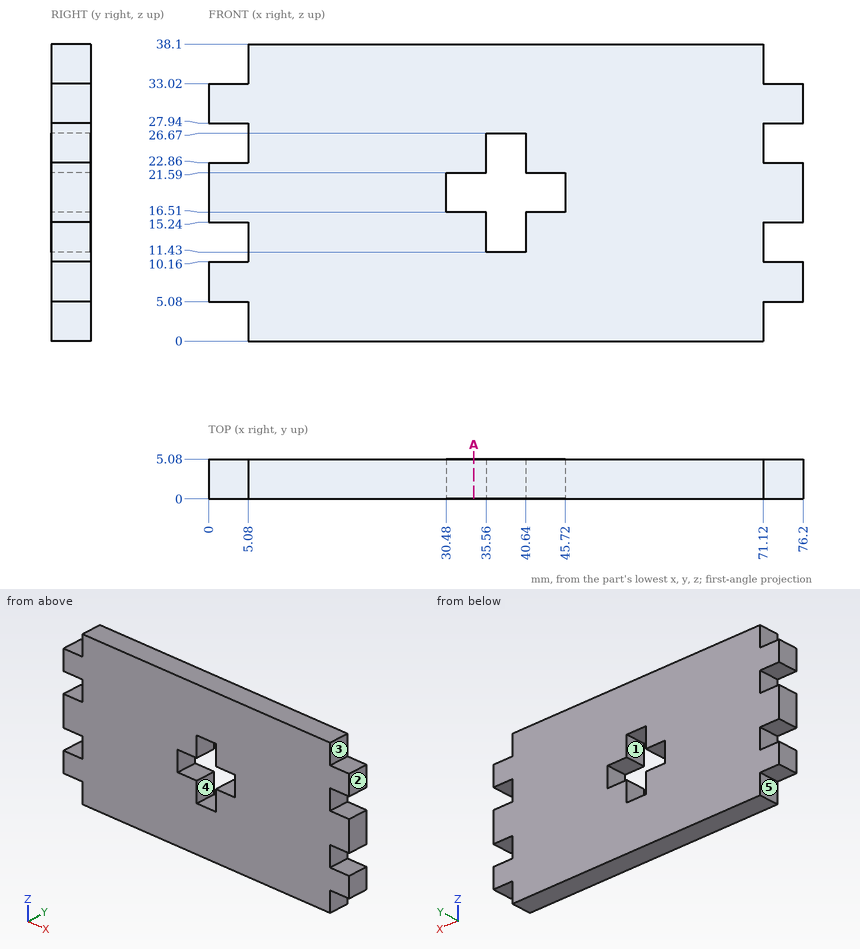
Drawing for the job (mm, zero at the part's lowest x, y, z). A direction names the side the tool comes from. Round coordinates to 2 decimals unless told otherwise and drop trailing zeros. Order: outer loops, then holes, each group sorted by start corner. A loop starts at its lowest first (then second) coordinate and runs counter-clockwise, first axis right, second up. Notation, with made-up numbers: (-18.75, -18.75) -> (-4.75, -18.75) arc R13 ccw to (-4.75, 4.25) -> close; hole circle Ø9 at (29.25, 66). An arc over 180 degrees is marked (long way). Write item = value, one per line. Start each with the question number.
(1) Cut at A-A, the plane x = 34. List the corners of the cut face in (y, z), then the cut area to 3 significant figures.
(2) Pin check, flat tips, straight feed: P1, Ø1.5, axis at y = 3, z = 3.5, coming from the -X side; P2, Ø1.5, axis at y = 1.5, z = 11.5, coming from the +X side; P3, Ø2.5, axis at x = 74, y = 2.5, coming from the -Z side. Stop position of each tip, or through.
(3) Probe line 1 (Z direction, x = 4, y = 3.95); line 2 (X direction, y = 3.5, z = 26); line 3 (X direction, y = 0.4, z = 16). List the from-to ranges inside material, lowest first. Write a range as [from, to].
(4) Pull direction Z, two halves, no side cores. Call the marked faces 4 and 5: released by +Z, released by -Z, zero draft, split by the parting line, or undercut.
(5) Which spindle directions (+Z, -Z, +X, -X, +Y, -Y) get a long thin tool onto all of the face, cutting with end or side? Do the marked faces 1, 2 and 3. Say none if no direction does.
Model answer:
q1.outline = (0, 0) -> (5.08, 0) -> (5.08, 16.51) -> (0, 16.51) -> close; (0, 21.59) -> (5.08, 21.59) -> (5.08, 38.1) -> (0, 38.1) -> close
q1.area = 168 mm2
q2.P1 = 5.08
q2.P2 = 71.12
q2.P3 = 5.08
q3.line_1 = [5.08, 10.16], [15.24, 22.86], [27.94, 33.02]
q3.line_2 = [5.08, 35.56], [40.64, 71.12]
q3.line_3 = [0, 35.56], [40.64, 76.2]
q4.face_4 = undercut
q4.face_5 = zero draft
q5.face_1 = +Y, -Y
q5.face_2 = +Z, -Z, +X, +Y, -Y
q5.face_3 = +Z, +X, +Y, -Y
